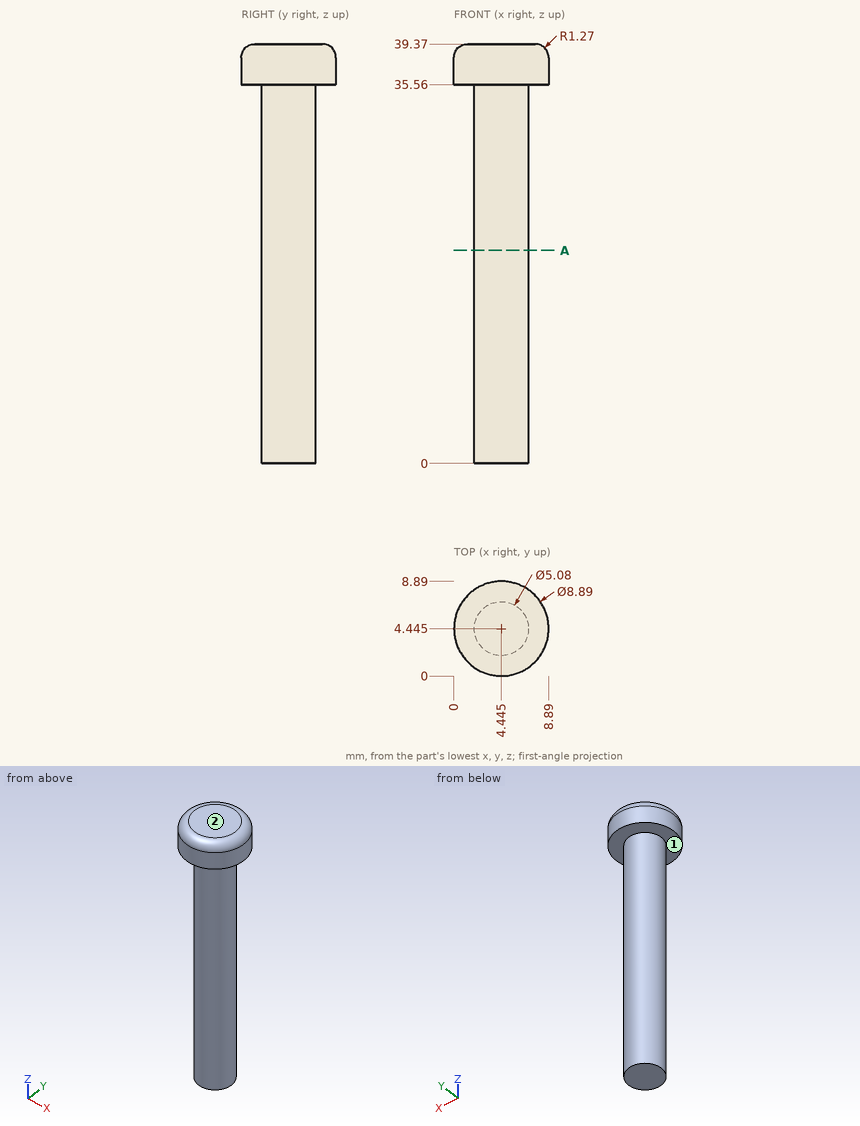
Design review of the part shown in the three views and the two pictorial views. Dimensions are in mm from the part's minimum x, y and z. A direction names the side the tool comes from. Give positions to 0.01 mm unless a question says otherwise; leave off trailing zeros. Loops run counter-clockwise (first coordinate to the right, second up) from the corner with the lowest first, then second, coordinate; pieces in that order, holes last. Notation, with made-up numbers: M 85.25,16.5 L 116.25,16.5 A10 ccw 116.25,27.5 Z; hole C -32.75,25.5 d5. An arc over 180 degrees is marked long. Answer as a JSON object with one key per item and string values. Group by question number.
Q1. Insertion check: P1, Ø1.5, axis at x = 2, z = 7, coming from the -Y side; P2, Ø1.5, axis at y = 4.5, z = 8, coming from the +X side (3 decimals). Each pin has a flat end and moves straight along its axis. Give the tip position at first contact, or say it passes through.
Q2. Add section A-A on z = 20. Give the boundary of the cut face in (x, y) (3 decimals), and give its area (3 significant figures).
Q3. Tool access review of the marked faces 1 and 2: name each direction out of +Z, -Z, +X, -X, +Y, -Y from which nothing blocks a thin tool from reaching the whole face with its end or side.
Q4. For probe 1 along Z at (x, y) = (5.5, 7.5); probe 2 along Y at (x, z) = (4.5, 27.5); probe 3 along Y at (x, z) = (6, 37.5), list the stretches that pass through material, from the lowest coordinate up. Write a range as [from, to].
Checked values:
{
 "1": {"P1": "y = 2.55", "P2": "x = 6.985"},
 "2": {"outline": "C 4.445,4.445 d5.08", "area": "20.3 mm²"},
 "3": {"face 1": "-Z", "face 2": "+Z, +X, -X, +Y, -Y"},
 "4": {"probe 1": "[35.56, 39.37]", "probe 2": "[1.91, 6.98]", "probe 3": "[0.28, 8.61]"}
}
